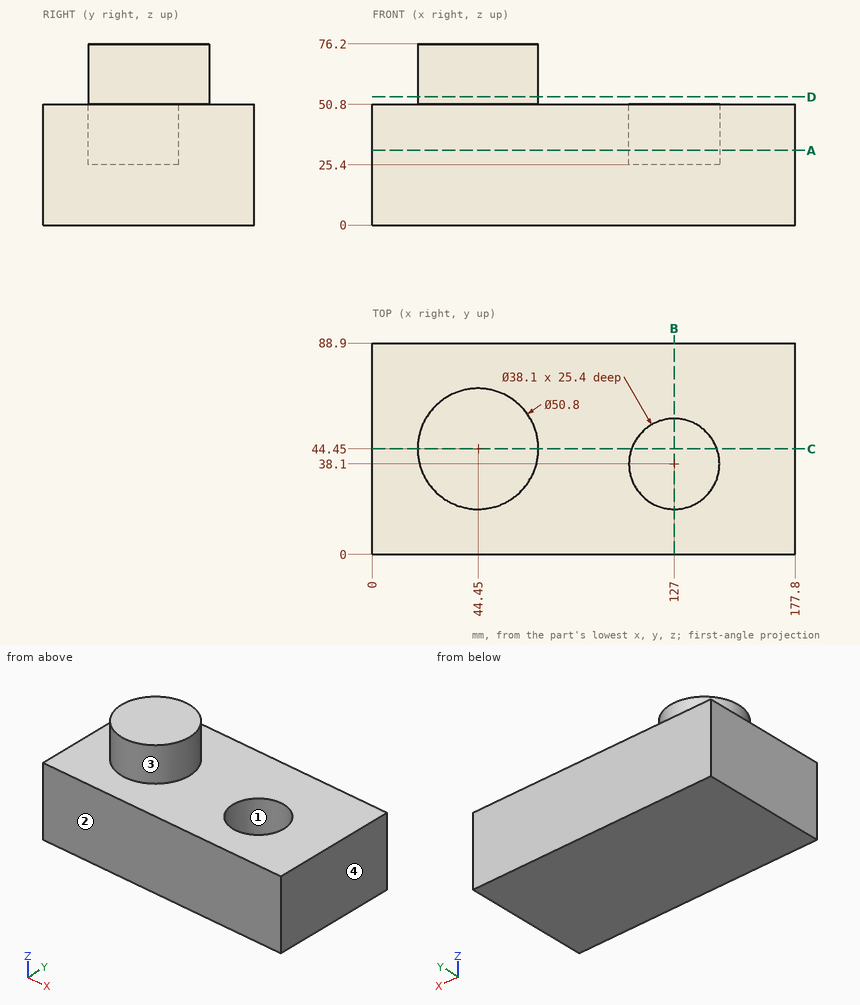
For this review, use the dimensioned drawing (mm, ordinates from the lowest corner) and the shaded views. Round coordinates to 2 decimals unless told otherwise and drop trailing zeros. Loops run counter-clockwise (first coordinate to the right, second up) from the corner with the lowest first, then second, coordinate; pieces in that order, holes last. Notation, with made-up numbers: (68.5, 85) -> (107.5, 85) arc R24 cw to (107.5, 121) -> close; hole circle Ø9 at (-6.75, -7.75). An arc over 180 degrees is marked (long way). Write item = value, one per line. Start each with the question number.
Item 1: Take a section at A-A on z = 31.5. Give the boundary of the cut face in (x, y), plus the area to 3 significant figures.
Item 2: Take a section at B-B on x = 127. Give the boundary of the cut face in (y, z).
Item 3: To check wall thickness, follow L1, parallel to Y at x = 127, z = 36; L2, parallel to Z at x = 93.5, y = 25; L3, parallel to X at y = 38, z = 37. State the ranges of each line that lie inside material, in increasing order.
Item 4: Take a section at C-C on y = 44.45. Give the boundary of the cut face in (x, z), plus the area to 3 significant figures.
Item 5: Mouldability with a two-part tool opening along X and no side actions: class the marked faces 1, 2, 3 and 4 as released by +X, released by -X, zero draft, split by the parting line, or undercut.
Item 6: Insertion check: pin 1 (1.5 mm diameter, centred on x = 140, y = 20.5, fed in from +Z); pin 2 (2 mm diameter, centred on x = 25, z = 52, fed in from -Y); pin 3 (12 mm diameter, centred on x = 21.5, z = 66.5, fed in from +Y); pin 4 (8 mm diameter, centred on x = 118.5, y = 76.5, fed in from -Z). Each pin has a flat end and moves straight along its axis. Give the tip position at first contact, or say it passes through.
Item 7: Take a section at D-D on z = 54. Give the boundary of the cut face in (x, y).
Result:
q1.outline = (0, 0) -> (177.8, 0) -> (177.8, 88.9) -> (0, 88.9) -> close; hole circle Ø38.1 at (127, 38.1)
q1.area = 14,700 mm²
q2.outline = (0, 0) -> (88.9, 0) -> (88.9, 50.8) -> (57.15, 50.8) -> (57.15, 25.4) -> (19.05, 25.4) -> (19.05, 50.8) -> (0, 50.8) -> close
q3.L1 = 0 to 19.05, 57.15 to 88.9
q3.L2 = 0 to 50.8
q3.L3 = 0 to 107.95, 146.05 to 177.8
q4.outline = (0, 0) -> (177.8, 0) -> (177.8, 50.8) -> (144.96, 50.8) -> (144.96, 25.4) -> (109.04, 25.4) -> (109.04, 50.8) -> (69.85, 50.8) -> (69.85, 76.2) -> (19.05, 76.2) -> (19.05, 50.8) -> (0, 50.8) -> close
q4.area = 9,410 mm²
q5.face_1 = undercut
q5.face_2 = zero draft
q5.face_3 = split by the parting line
q5.face_4 = released by +X
q6.pin_1 = 50.8
q6.pin_2 = 26.99
q6.pin_3 = 63.37
q6.pin_4 = 0
q7.outline = circle Ø50.8 at (44.45, 44.45)
